Work out the finished part from the listing and answer in its coordinate system (mm). A direction names the side the tool comes from. Give positions to 0.01 mm unless a question says otherwise; leave off trailing zeros. Write each loop counter-clockwise with the first axis right and the second up, starting at its lowest first coordinate (ties: lowest second). Pieces come first, ordered by that corner, then holes.
1) Given pin 1 Ø3 at (y, z) = (1, 4) entering from -X; pin 2 Ø3 at (x, z) = (1, 4) entering from -Y; pin 3 Ø0.8 at (x, z) = (-1, 5.5) entering from +Y, each flat-ended and moving along its own axis, determine where each tip first touches the part or whether it passes through.
2) Find section B-B (y = 4). Determine the outline of the cut face in (x, z), plus the area to 3 significant figures.
3) Find section A-A (z = 5.6). Determine the outline of the cut face in (x, y).
4) Find section D-D (y = 0.5). Determine the outline of the cut face in (x, z), plus the area to 3 significant figures.
5) Straight lines are drawn through the part: probe 1 along Z at (x, y) = (6.75, 0.5); probe 2 along X at (y, z) = (-4, 3.5); probe 3 along X at (y, z) = (2.5, 5.6). For each, find the intervals that lie inside material, in ascending order.
6) A tool of negligible diameter and unlimited length cuts with its end or side. For faces 1 (the face through (6.16, -6.18, 3.97)), 2 (the face through (0, -6.55, 4)), 3 (the face through (-6.18, -6.16, 3.97)), 4 (the face through (-7, 0, 2)), 5 (the face through (-6.55, 0, 4)), from which of +Z, -Z, +X, -X, +Y, -Y can it reach the whole face along a straight path? Write none if from no direction.
```python
from build123d import *

# Parameters (mm, degrees)
F0_W     = 15.5
F0_H     = 15.5
F1_DEPTH = 2
F2_DEPTH = 6
F3_DEPTH = 5.25


with BuildPart() as f1:
    # F0 (on Top) → F1 (new body)
    with BuildSketch(Plane.XY):
        Rectangle(F0_W, F0_H)
        with BuildLine():
            Line((-6.549937, -5.249806), (-6.549937, 5.250194))
            ThreePointArc((-6.549937, 5.250194), (-6.169176, 6.169433), (-5.249937, 6.550194))
            Line((-5.249937, 6.550194), (5.250063, 6.550194))
            ThreePointArc((5.250063, 6.550194), (6.169302, 6.169433), (6.550063, 5.250194))
            Line((6.550063, 5.250194), (6.550063, -5.249806))
            ThreePointArc((6.550063, -5.249806), (6.169302, -6.169045), (5.250063, -6.549806))
            Line((5.250063, -6.549806), (-5.249937, -6.549806))
            ThreePointArc((-5.249937, -6.549806), (-6.169176, -6.169045), (-6.549937, -5.249806))
        make_face(mode=Mode.SUBTRACT)
    extrude(amount=F1_DEPTH)

    # F0 (on Top) → F2 (join)
    with BuildSketch(Plane.XY):
        with BuildLine():
            ThreePointArc((-5.249937, 6.550194), (-6.169176, 6.169433), (-6.549937, 5.250194))
            Line((-6.549937, 5.250194), (-6.549937, -5.249806))
            ThreePointArc((-6.549937, -5.249806), (-6.169176, -6.169045), (-5.249937, -6.549806))
            Line((-5.249937, -6.549806), (5.250063, -6.549806))
            ThreePointArc((5.250063, -6.549806), (6.169302, -6.169045), (6.550063, -5.249806))
            Line((6.550063, -5.249806), (6.550063, 5.250194))
            ThreePointArc((6.550063, 5.250194), (6.169302, 6.169433), (5.250063, 6.550194))
            Line((5.250063, 6.550194), (-5.249937, 6.550194))
        make_face()
        Polygon((1.24317, -3.46653), (0.205601, -3.46653), (0.205601, 2.567623), (-1.243169, 2.567623), (-0.803279, 3.46653), (1.24317, 3.46653), align=None, mode=Mode.SUBTRACT)
    extrude(amount=F2_DEPTH)

    # F0 (on Top) → F3 (join)
    with BuildSketch(Plane.XY):
        Polygon((0.205601, 2.567623), (0.205601, -3.46653), (1.24317, -3.46653), (1.24317, 3.46653), (-0.803279, 3.46653), (-1.243169, 2.567623), align=None)
    extrude(amount=F3_DEPTH)


solid = f1.part
```
Results:
1. pin 1: stops at x = -6.55
1. pin 2: stops at y = -6.55
1. pin 3: stops at y = 6.55
2. outline: (-7.75, 0) - (7.75, 0) - (7.75, 2) - (6.55, 2) - (6.55, 6) - (-6.55, 6) - (-6.55, 2) - (-7.75, 2) - close
2. area: 83.4 mm2
3. outline: (-6.55, -5.25) arc R1.3 ccw to (-5.25, -6.55) - (5.25, -6.55) arc R1.3 ccw to (6.55, -5.25) - (6.55, 5.25) arc R1.3 ccw to (5.25, 6.55) - (-5.25, 6.55) arc R1.3 ccw to (-6.55, 5.25) - close; hole (-1.24, 2.57) - (0.21, 2.57) - (0.21, -3.47) - (1.24, -3.47) - (1.24, 3.47) - (-0.8, 3.47) - close
4. outline: (-7.75, 0) - (7.75, 0) - (7.75, 2) - (6.55, 2) - (6.55, 6) - (1.24, 6) - (1.24, 5.25) - (0.21, 5.25) - (0.21, 6) - (-6.55, 6) - (-6.55, 2) - (-7.75, 2) - close
4. area: 82.6 mm2
5. probe 1: z = 0 to 2
5. probe 2: x = -6.55 to 6.55
5. probe 3: x = -6.55 to 0.21, 1.24 to 6.55
6. face 1: +Z, +X, -Y
6. face 2: +Z, +X, -X, -Y
6. face 3: +Z, -X, -Y
6. face 4: +Z
6. face 5: +Z, -X, +Y, -Y
